Can you work these out from the model? Positions are in its coordinate system, mm. Face numbers are marked on the shaded views. A direction names the side the tool comes from. Give positions to 0.01 mm unless a question says otherwise; leave off trailing zeros. Order: outer loops, then holes, each group sorted by start corner. A loop starts at its lowest first (then second) coordinate and runs counter-clockwise, first axis right, second up. Notation, with made-up numbers: (19, 33.25) - (70, 33.25) arc R20 ccw to (70, 49.25) - close; hole circle Ø10 at (71.25, -32.5). An arc over 180 degrees is marked (long way). Use one line per item in the form item = value. Start each with the question number.
1) For pin 1 (12 mm diameter, centred on x = -15, y = -19.5, fed in from +Z); pin 2 (10 mm diameter, centred on y = -21, z = 16, fed in from -X); pin 3 (11 mm diameter, centred on x = -12, y = -8.5, fed in from -Z), each with a flat end and sliding along its axis, tell me the tip position at first contact or that it passes through.
2) Suppose I cut it at C-C, the plane x = -4.5. Write out the boundary of the cut face in (y, z).
3) Suppose I cut it at D-D, the plane x = 42. Write out the boundary of the cut face in (y, z), and give its area (3 significant figures).
4) Suppose I cut it at B-B, the plane y = -5.5. Write out the boundary of the cut face in (x, z).
5) Please list where these lines run through material, in increasing order: probe 1 along Z at (x, y) = (26, -16.5); probe 2 along X at (y, z) = (-25, 59.5); probe 3 along X at (y, z) = (-9.5, 50).
6) We'd pull the mould along X, two halves only. Please class the marked faces 1, 2 and 3: released by +X, released by -X, zero draft, split by the parting line, or undercut.
7) Which directions (+Z, -Z, +X, -X, +Y, -Y) give clear straight access to the entire face, cutting with the end or side of a thin tool? Please do the marked faces 4, 5 and 6.
8) Suppose I cut it at A-A, the plane x = 26. Write out the boundary of the cut face in (y, z), and give its area (3 significant figures).
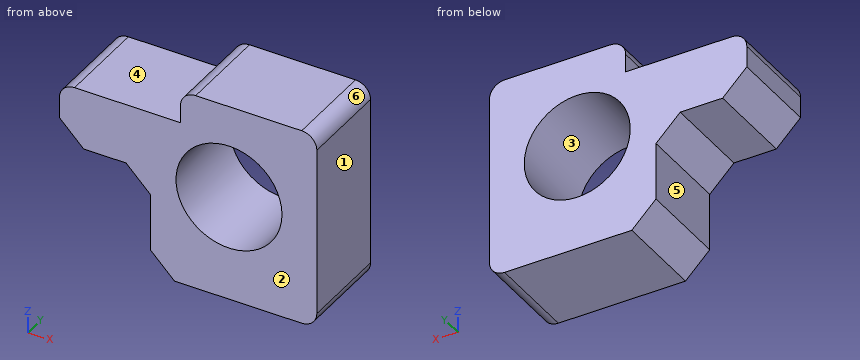
```python
from build123d import *

# Parameters (mm, degrees)
F0_R     = 17.5
F1_DEPTH = 30
F2_R     = 5
F3_SIZE  = 8


with BuildPart() as f1:
    # F0 (on Front) → F1 (new body)
    with BuildSketch(Plane.XZ):
        Polygon((0, 35), (0, 0), (55, 0), (55, 66), (10, 66), (10, 55), (-30, 55), (-30, 35), align=None)
        with Locations((26, 35)):
            Circle(F0_R, mode=Mode.SUBTRACT)
    extrude(amount=F1_DEPTH)

    # F2
    f2_edges = [f1.edges().sort_by_distance(p)[0] for p in [
        (10, -15, 66),
        (55, -15, 66),
        (55, -15, 0),
        (-30, -15, 55),
    ]]
    fillet(f2_edges, radius=F2_R)

    # F3
    f3_edges = [f1.edges().sort_by_distance(p)[0] for p in [
        (0, -15, 35),
        (-30, -15, 35),
        (0, -15, 0),
    ]]
    chamfer(f3_edges, length=F3_SIZE)


solid = f1.part
```
Result sheet:
q1.pin_1 = 55
q1.pin_2 = 0
q1.pin_3 = 33.5
q2.outline = (-30, 31.5) - (0, 31.5) - (0, 55) - (-30, 55) - close
q3.outline = (-30, 0) - (0, 0) - (0, 27.91) - (-30, 27.91) - close; (-30, 42.09) - (0, 42.09) - (0, 66) - (-30, 66) - close
q3.area = 1,550 mm²
q4.outline = (-30, 43) - (-22, 35) - (-8, 35) - (0, 27) - (0, 8) - (8, 0) - (50, 0) arc R5 ccw to (55, 5) - (55, 61) arc R5 ccw to (50, 66) - (15, 66) arc R5 ccw to (10, 61) - (10, 55) - (-25, 55) arc R5 ccw to (-30, 50) - close; hole circle Ø35 at (26, 35)
q5.probe_1 = 0 to 17.5, 52.5 to 66
q5.probe_2 = 10 to 55
q5.probe_3 = -30 to 16.99, 35.01 to 55
q6.face_1 = released by +X
q6.face_2 = zero draft
q6.face_3 = undercut
q7.face_4 = +Z, -X, +Y, -Y
q7.face_5 = -Z, -X, +Y, -Y
q7.face_6 = +Z, +X, +Y, -Y
q8.outline = (-30, 0) - (0, 0) - (0, 17.5) - (-30, 17.5) - close; (-30, 52.5) - (0, 52.5) - (0, 66) - (-30, 66) - close
q8.area = 930 mm²
